from build123d import *

# Parameters (mm, degrees)
BOSS_EXTRUDE1_DEPTH = 6.35
SKETCH2_R           = 3.175
CUT_EXTRUDE1_DEPTH  = 302.34078715
CUT_EXTRUDE2_DEPTH  = 302.34078715
FILLET1_R           = 6.35


with BuildPart() as part:
    # Sketch1 → Boss-Extrude1 (new, symmetric)
    with BuildSketch(Plane(origin=(0, 0, 0), x_dir=(1, 0, 0), z_dir=(0, 1, 0))):
        Polygon((-266.7, -139.7), (266.7, -139.7), (266.7, 139.7), (170.18, 139.7), (146.939, 88.9), (-108.237741638, 88.9), (-169.2275, 139.7), (-266.7, 139.7), align=None)
    extrude(amount=BOSS_EXTRUDE1_DEPTH, both=True)

    # Sketch2 → Cut-Extrude1 (cut, through all)
    with BuildSketch(Plane(origin=(0, 6.35, 0), x_dir=(1, 0, 0), z_dir=(0, 1, 0))):
        with Locations(Location((81.4832, 6.2484, 0), (0, 0, 270))):
            Circle(SKETCH2_R)
        with Locations(Location((81.4832, 32.4104, 0), (0, 0, 270))):
            Circle(SKETCH2_R)
        with Locations(Location((57.1627, 32.4104, 0), (0, 0, 270))):
            Circle(SKETCH2_R)
        with Locations(Location((32.8422, 32.4104, 0), (0, 0, 270))):
            Circle(SKETCH2_R)
        with Locations(Location((32.8422, 6.2484, 0), (0, 0, 270))):
            Circle(SKETCH2_R)
        with Locations(Location((57.1627, 6.2484, 0), (0, 0, 270))):
            Circle(SKETCH2_R)
    extrude(amount=-CUT_EXTRUDE1_DEPTH, mode=Mode.SUBTRACT)

    # Sketch3 → Cut-Extrude2 (cut, through all)
    with BuildSketch(Plane(origin=(0, 6.35, 0), x_dir=(1, 0, 0), z_dir=(0, 1, 0))):
        Polygon((-266.7, 34.925), (-146.05, -139.7), (-266.7, -139.7), align=None)
    cut_extrude2 = extrude(amount=-CUT_EXTRUDE2_DEPTH, mode=Mode.SUBTRACT)

    # Mirror1: Cut-Extrude2 across plane
    add(cut_extrude2.mirror(Plane(origin=(0, 0, 0), x_dir=(0, 0, 1), z_dir=(1, 0, 0))), mode=Mode.SUBTRACT)

    # Fillet1
    fillet1_edges = [part.edges().sort_by_distance(p)[0] for p in [
        (170.18, 0, -139.7),
        (266.7, 0, -139.7),
        (-266.7, 0, -34.925),
        (-146.05, 0, 139.7),
        (266.7, 0, -34.925),
        (146.05, 0, 139.7),
    ]]
    fillet(fillet1_edges, radius=FILLET1_R)


solid = part.part
CAD build for the part. Positions are in the model's coordinates, mm. A direction names the side the tool comes from. Round coordinates to 2 decimals unless told otherwise and drop trailing zeros. Order: outer loops, then holes, each group sorted by start corner. A loop starts at its lowest first (then second) coordinate and runs counter-clockwise, first axis right, second up. Notation, with made-up numbers: (5, 80.5) - (30, 80.5) arc R26 cw to (30, 117.5) - close; hole circle Ø1 at (-18, -30). An arc over 180 degrees is marked (long way). Return JSON: item names as keys, results as strings.
(1) Pull direction X, two halves, no side cores. Call faces 1 (the face through (-266.7, 0, -89)), 2 (the face through (-217, 0, -139.7)), 3 (the face through (207.58, 0.09, 50.64)), 4 (the face through (-138.306, 0.089, -113.944)): +X half, -X half, draft (parallel to the pull), parting line (faces both ways), or undercut.
Answer key:
{"face 1": "-X half", "face 2": "draft", "face 3": "+X half", "face 4": "undercut"}
(2) Cut at A-A (z = -112). Give the cut face in (x, y).
Answer key:
{"outline": "(-266.7, -6.35) - (-135.97, -6.35) - (-135.97, 6.35) - (-266.7, 6.35) - close; (157.51, -6.35) - (266.7, -6.35) - (266.7, 6.35) - (157.51, 6.35) - close"}
(3) Cut at B-B (y = -2). State how many separate pieces and enclosed holes the cut face has, then the cut area to 3 significant figures.
Answer key:
{"separate pieces": "1", "enclosed holes": "6", "area": "113,000 mm^2"}
(4) Cut at D-D (z = 59). Give the cut face in (x, y), then the cut area to 3 significant figures.
Answer key:
{"outline": "(-201.81, -6.35) - (201.81, -6.35) - (201.81, 6.35) - (-201.81, 6.35) - close", "area": "5,130 mm^2"}
(5) Pin check, flat tips, straight feed: pin 1 Ø5 at (x, z) = (32.84, -6.25) entering from +Y; pin 2 Ø4 at (y, z) = (-0.5, -24.5) entering from -X; pin 3 Ø4 at (x, y) = (-55, 3) entering from -Z; pin 4 Ø2 at (y, z) = (-1, 30.5) entering from -X. Stop position of each tip, or through.
Answer key:
{"pin 1": "passes through", "pin 2": "stops at x = -260.88", "pin 3": "stops at z = -88.9", "pin 4": "stops at x = -222.19"}
(6) Wall check: probe 1 along Z at (x, y) = (60, -4.25); probe 2 along Z at (x, y) = (136, -0.25); probe 3 along Z at (x, y) = (197, -2.5). Give the ranges that are in metal, low to high. Write a range as from..to.
Answer key:
{"probe 1": "z = -88.9..-33.84, -30.99..-7.67, -4.82..139.7", "probe 2": "z = -88.9..139.7", "probe 3": "z = -139.7..65.96"}
(7) Tool access for faces 5 (the face through (157.862, 0.089, -112.776)), 6 (the face through (266.7, 0, -84)): list every direction of +Z, -Z, +X, -X, +Y, -Y with a clear straight run to the whole face (end or side of a thin tool).
Answer key:
{"face 5": "-Z, +Y, -Y", "face 6": "+Z, -Z, +X, +Y, -Y"}
(8) Cut at C-C (x = -62). Give the cut face in (y, z).
Answer key:
{"outline": "(-6.35, -88.9) - (6.35, -88.9) - (6.35, 139.7) - (-6.35, 139.7) - close"}
